Source: CAD feature listing. Evaluate the final solid. Frame: model axes, mm. Face numbers are marked on the shaded views. Give positions to 0.01 mm unless a question says otherwise; leave off trailing zeros. Write each loop counter-clockwise with the first axis right and the second up, starting at its lowest first coordinate (ties: lowest second). Pieces come first, ordered by that corner, then holes. Notation, with made-up numbers: M -36,82.5 L -31,82.5 A17 ccw -31,105.5 Z; hole C 79,-0.5 d5. An arc over 180 degrees is marked long. Return JSON: item names as keys, results as strings.
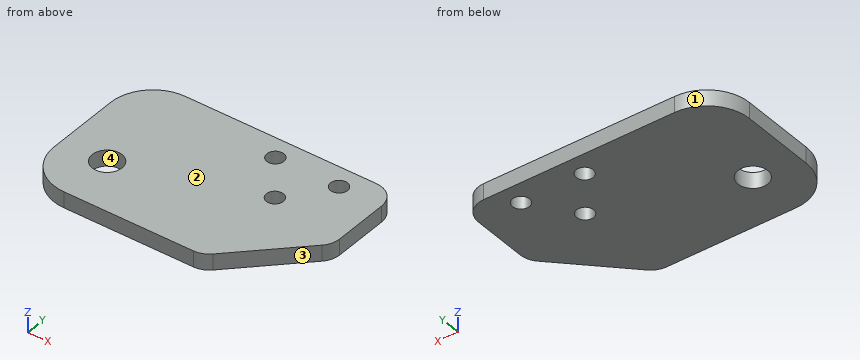
```python
from build123d import *

# Parameters (mm, degrees)
SKETCH070_W     = 48
SKETCH070_H     = 30
SKETCH070_R     = 2.8
SKETCH070_R_2   = 1.6
PAD025_DEPTH    = 3
CHAMFER029_SIZE = 14
FILLET015_R     = 8
FILLET016_R     = 4


with BuildPart() as part:
    # Sketch070 → Pad025 (new body)
    with BuildSketch(Plane.XY):
        with Locations((4, 5)):
            Rectangle(SKETCH070_W, SKETCH070_H)
        with Locations((-11.5, 0)):
            Circle(SKETCH070_R, mode=Mode.SUBTRACT)
        with Locations((8, 16)):
            Circle(SKETCH070_R_2, mode=Mode.SUBTRACT)
        with Locations((20, 16)):
            Circle(SKETCH070_R_2, mode=Mode.SUBTRACT)
        with Locations((14, 8)):
            Circle(SKETCH070_R_2, mode=Mode.SUBTRACT)
    extrude(amount=-PAD025_DEPTH)

    # Chamfer029
    chamfer029_edges = [part.edges().sort_by_distance(p)[0] for p in [
        (28, -10, -1.5),
    ]]
    chamfer(chamfer029_edges, length=CHAMFER029_SIZE)

    # Fillet015
    fillet015_edges = [part.edges().sort_by_distance(p)[0] for p in [
        (-20, -10, -1.5),
        (-20, 20, -1.5),
    ]]
    fillet(fillet015_edges, radius=FILLET015_R)

    # Fillet016
    fillet016_edges = [part.edges().sort_by_distance(p)[0] for p in [
        (28, 20, -1.5),
        (28, 4, -1.5),
        (14, -10, -1.5),
    ]]
    fillet(fillet016_edges, radius=FILLET016_R)


with BuildPart() as part_1:
    # Body014 placement: moved
    add(part.part.moved(Location((108, -82, -3.7))))


solid = part_1.part
```
1) Cut plane C-C, the plane z = -5.1. Return the cut outline in (x, y), then the cut area to 3 significant figures.
Numbers:
{"outline": "M 88,-84 A8 ccw 96,-92 L 120.34,-92 A4 ccw 123.17,-90.83 L 134.83,-79.17 A4 ccw 136,-76.34 L 136,-66 A4 ccw 132,-62 L 96,-62 A8 ccw 88,-70 Z; hole C 96.5,-82 d5.6; hole C 116,-66 d3.2; hole C 122,-74 d3.2; hole C 128,-66 d3.2", "area": "1,260 mm²"}
2) Cut plane B-B, the plane x = 116. Return the cut outline in (y, z).
Numbers:
{"outline": "M -92,-6.7 L -67.6,-6.7 L -67.6,-3.7 L -92,-3.7 Z; M -64.4,-6.7 L -62,-6.7 L -62,-3.7 L -64.4,-3.7 Z"}
3) Cut plane D-D, the plane y = -66.5. Return the cut outline in (x, z).
Numbers:
{"outline": "M 88.81,-6.7 L 114.48,-6.7 L 114.48,-3.7 L 88.81,-3.7 Z; M 117.52,-6.7 L 126.48,-6.7 L 126.48,-3.7 L 117.52,-3.7 Z; M 129.52,-6.7 L 136,-6.7 L 136,-3.7 L 129.52,-3.7 Z"}
4) Draft query along X for the marked faces 1, 2, 3 and 4. Return one class per face: released by +X, released by -X, zero draft, split by the parting line, or undercut.
Numbers:
{"face 1": "released by -X", "face 2": "zero draft", "face 3": "released by +X", "face 4": "undercut"}
5) Cut plane A-A, the plane y = -82. Return the cut outline in (x, z).
Numbers:
{"outline": "M 88,-6.7 L 93.7,-6.7 L 93.7,-3.7 L 88,-3.7 Z; M 99.3,-6.7 L 132,-6.7 L 132,-3.7 L 99.3,-3.7 Z"}
6) Line query: line 1 (Y direction, x = 116, z = -4.85); line 2 (X direction, y = -66, z = -5.35); line 3 (Y direction, x = 96.5, z = -5.5). Output: solid intervals per line, ascending. Write a range as [from, to].
Numbers:
{"line 1": "y = [-92, -67.6], [-64.4, -62]", "line 2": "x = [89.07, 114.4], [117.6, 126.4], [129.6, 136]", "line 3": "y = [-92, -84.8], [-79.2, -62]"}
7) Contact query for a flat-ended pin moving along its axis: pin 1 Ø9 at (x, y) = (96.5, -82) entering from -Z. Output: stop coordinate, or through.
Numbers:
{"pin 1": "stops at z = -6.7"}
